from build123d import *

# Parameters (mm, degrees)
SKETCH_1_R          = 3.5
EXTRUDE_1_DEPTH     = 3.5
CUT_EXTRUDE_1_DEPTH = 2
SKETCH_3_R          = 2
EXTRUDE_2_DEPTH     = 23
SKETCH_4_R          = 1.5
EXTRUDE_3_DEPTH     = 6


with BuildPart() as part:
    # 草图1 → 凸台-拉伸1 (new body)
    with BuildSketch(Plane.XY):
        Circle(SKETCH_1_R)
    extrude(amount=EXTRUDE_1_DEPTH)

    # 草图2 → 切除-拉伸1 (cut)
    with BuildSketch(Plane.XY.offset(3.5)):
        Polygon((0.893639487, 1.483714416), (-0.838114632, 1.515771705), (-1.731754119, 0.03205729), (-0.893639487, -1.483714416), (0.838114632, -1.515771705), (1.731754119, -0.03205729), align=None)
    extrude(amount=-CUT_EXTRUDE_1_DEPTH, mode=Mode.SUBTRACT)

    # 草图3 → 凸台-拉伸2 (add)
    with BuildSketch(Plane(origin=(0, 0, 0), x_dir=(-1, 0, 0), z_dir=(0, 0, -1))):
        with Locations(Location((0, 0, 0), (0, 0, 180))):
            Circle(SKETCH_3_R)
    extrude(amount=EXTRUDE_2_DEPTH)

    # 草图4 → 凸台-拉伸3 (add)
    with BuildSketch(Plane(origin=(0, 0, -23), x_dir=(-1, 0, 0), z_dir=(0, 0, -1))):
        Circle(SKETCH_4_R)
    extrude(amount=EXTRUDE_3_DEPTH)


solid = part.part
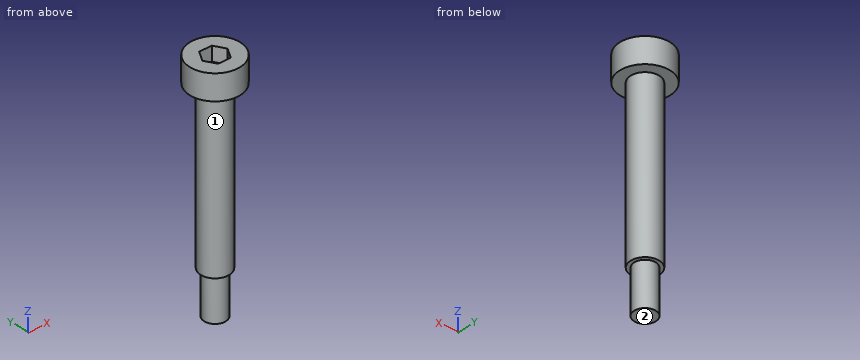
Geometry: final body of the model. Coordinates: model frame, mm. Face numbers are marked on the shaded views. A direction names the side the tool comes from. Round coordinates to 2 decimals unless told otherwise and drop trailing zeros. Order: outer loops, then holes, each group sorted by start corner. A loop starts at its lowest first (then second) coordinate and runs counter-clockwise, first axis right, second up. Notation, with made-up numbers: (84, -28.5) -> (129, -28.5) arc R19 cw to (129, -9.5) -> close; hole circle Ø9 at (59.25, -9.75). An arc over 180 degrees is marked (long way). Put each result on its own line as item: value. Start each with the question number.
Q1. Section B-B on x = 0. Return the cut outline in (y, z), and give its area (3 significant figures).
Q2. Line query: probe 1 along Z at (x, y) = (1.75, 0.25); probe 2 along Z at (x, y) = (-1.25, 0.5); probe 3 along Y at (x, z) = (0, -2.5). Output: solid intervals per line, ascending.
Q3. Section A-A on y = 1. Return the cut outline in (x, z), and give its area (3 significant figures).
Q4. Section C-C on z = -0.5. Return the cut outline in (x, y).
Q5. Reachability of the marked faces 1 and 2 from +Z, -Z, +X, -X, +Y, -Y: full face, straight path, thin tool, end or side. Return the list, or none.
Q6. First-contact query: pin 1 (4 mm diameter, centred on x = 2.5, z = -10.5, fed in from -Y); pin 2 (1.5 mm diameter, centred on y = -1.5, z = -0.5, fed in from +X); pin 3 (2 mm diameter, centred on y = 0.5, z = -4, fed in from -X). Flat tips, straight axial feed; report the tip coordinate or a pass-through.
Ans:
1. outline: (-3.5, 0) -> (-2, 0) -> (-2, -23) -> (-1.5, -23) -> (-1.5, -29) -> (1.5, -29) -> (1.5, -23) -> (2, -23) -> (2, 0) -> (3.5, 0) -> (3.5, 3.5) -> (1.5, 3.5) -> (1.5, 1.5) -> (-1.5, 1.5) -> (-1.5, 3.5) -> (-3.5, 3.5) -> close
1. area: 128 mm2
2. probe 1: z = -23 to 3.5
2. probe 2: z = -29 to 1.5
2. probe 3: y = -2 to 2
3. outline: (-3.35, 0) -> (-1.73, 0) -> (-1.73, -23) -> (-1.12, -23) -> (-1.12, -29) -> (1.12, -29) -> (1.12, -23) -> (1.73, -23) -> (1.73, 0) -> (3.35, 0) -> (3.35, 3.5) -> (1.16, 3.5) -> (1.16, 1.5) -> (-1.15, 1.5) -> (-1.15, 3.5) -> (-3.35, 3.5) -> close
3. area: 112 mm2
4. outline: circle Ø4 at (0, 0)
5. face 1: -Z
5. face 2: -Z, +X, -X, +Y, -Y
6. pin 1: stops at y = -1.94
6. pin 2: stops at x = 3.37
6. pin 3: stops at x = -2
